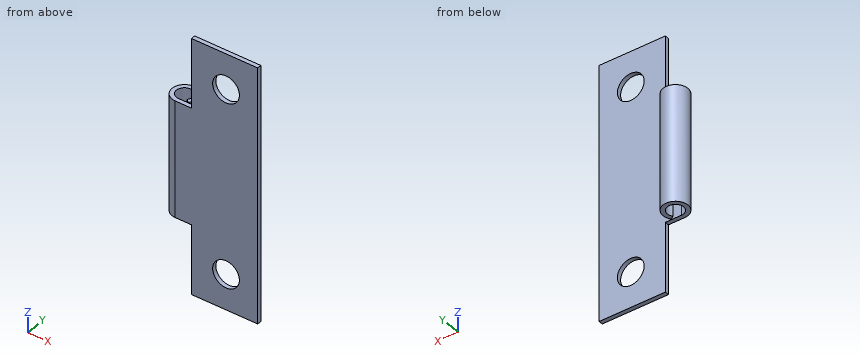
```python
from build123d import *

# Parameters (mm, degrees)
BOSS_EXTRUDE1_DEPTH     = 36
SKETCH2_R               = 1.9
CUT_EXTRUDE1_DEPTH      = 39.543989963
CUT_EXTRUDE2_DEPTH      = 39.543989963
CUT_EXTRUDE2_DEPTH_BACK = 39.543989963
SKETCH3_W               = 6.778348146
SKETCH3_H               = 10.807071142
SKETCH3_W_2             = 8.880524156
SKETCH3_H_2             = 10.732304286


with BuildPart() as part:
    # Sketch1 → Boss-Extrude1 (new body)
    with BuildSketch(Plane.XY):
        with BuildLine():
            Line((0, 0), (0, 0.6))
            Line((0, 0.6), (-11.712138102, 0.6))
            ThreePointArc((-11.712138102, 0.6), (-12.215259426, 2.784102961), (-10.807304622, 1.040227943))
            Line((-10.807304622, 1.040227943), (-10.335217589, 0.669912086))
            ThreePointArc((-10.335217589, 0.669912086), (-12.477757508, 3.32363494), (-11.712138102, 0))
            Line((-11.712138102, 0), (0, 0))
        make_face()
    extrude(amount=BOSS_EXTRUDE1_DEPTH)

    # Sketch2 → Cut-Extrude1 (cut, through all)
    with BuildSketch(Plane(origin=(0, 0.6, 0), x_dir=(1, 0, 0), z_dir=(0, 1, 0))):
        with Locations(Location((-4.5, -5, 0), (0, 0, 180))):
            Circle(SKETCH2_R)
        with Locations(Location((-4.5, -31, 0), (0, 0, 180))):
            Circle(SKETCH2_R)
    extrude(amount=-CUT_EXTRUDE1_DEPTH, mode=Mode.SUBTRACT)

    # Sketch3 → Cut-Extrude2 (cut, two sides: drawn at the far end of the back side and taken through both)
    with BuildSketch(Plane(origin=(0, 0.6, 0), x_dir=(1, 0, 0), z_dir=(0, 1, 0)).offset(-CUT_EXTRUDE2_DEPTH_BACK)):
        with Locations((-12.789174073, -4.396464429)):
            Rectangle(SKETCH3_W, SKETCH3_H)
        with Locations((-13.840262078, -31.566152143)):
            Rectangle(SKETCH3_W_2, SKETCH3_H_2)
    extrude(amount=CUT_EXTRUDE2_DEPTH + CUT_EXTRUDE2_DEPTH_BACK, mode=Mode.SUBTRACT)


solid = part.part
```
Work out the finished part from the listing and answer in its coordinate system (mm). Give positions to 0.01 mm unless a question says otherwise; leave off trailing zeros. Loops run counter-clockwise (first coordinate to the right, second up) from the corner with the lowest first, then second, coordinate; pieces in that order, holes last. Notation, with made-up numbers: (-24.75, -4.75) -> (-14.75, -4.75) arc R18 cw to (-14.75, 2.25) -> close; hole circle Ø9 at (88.5, -24.75). An arc over 180 degrees is marked (long way). Write item = value, one per line. Start each with the question number.
(1) Find section A-A on y = 1.75. Give the vertices of the cut face in (x, z), and give its area (3 significant figures).
(2) Find section C-C on z = 13. Give the vertices of the cut face in (x, y), and give its area (3 significant figures).
(3) Given pin 1 Ø1.5 at (x, y) = (-10.5, 1.5) entering from +Z; pin 2 Ø3 at (x, z) = (-4.5, 22) entering from -Y; pin 3 Ø1.5 at (y, z) = (2, 24.5) entering from +X; pin 4 Ø0.7 at (y, z) = (0.5, 4.5) entering from -X, each flat-ended and moving along its own axis, determine where each tip first touches the part or whether it passes through.
(4) Find the intervals of material crossed by probe 1 along Z at (x, y) = (-4.5, 0.4); probe 2 along X at (y, z) = (1.75, 22.5); probe 3 along Y at (x, z) = (-6.5, 29), in increasing order. Write a range as from..to.
(5) Find section B-B on z = 31. Give the vertices of the cut face in (x, y).
(6) Find section D-D on x = -8.5. Give the vertices of the cut face in (y, z).
From the geometry:
q1.outline = (-13.46, 9.8) -> (-12.86, 9.8) -> (-12.86, 26.2) -> (-13.46, 26.2) -> close; (-10.56, 9.8) -> (-9.96, 9.8) -> (-9.96, 26.2) -> (-10.56, 26.2) -> close
q1.area = 19.7 mm^2
q2.outline = (-11.71, 0) -> (0, 0) -> (0, 0.6) -> (-11.71, 0.6) arc R1.15 cw (long way) to (-10.81, 1.04) -> (-10.34, 0.67) arc R1.75 ccw (long way) to start
q2.area = 11.7 mm^2
q3.pin_1 = 26.2
q3.pin_2 = 0
q3.pin_3 = -9.96
q3.pin_4 = -9.4
q4.probe_1 = 0..3.1, 6.9..29.1, 32.9..36
q4.probe_2 = -13.46..-12.86, -10.56..-9.96
q4.probe_3 = 0..0.6
q5.outline = (-9.4, 0) -> (-6.4, 0) -> (-6.4, 0.6) -> (-9.4, 0.6) -> close; (-2.6, 0) -> (0, 0) -> (0, 0.6) -> (-2.6, 0.6) -> close
q6.outline = (0, 0) -> (0.6, 0) -> (0.6, 36) -> (0, 36) -> close
